from build123d import *

# Parameters (mm, degrees)
SKETCH1_R           = 5.55625
BOSS_EXTRUDE1_DEPTH = 3.175
SKETCH2_R           = 2.3876
CUT_EXTRUDE1_DEPTH  = 7.35


with BuildPart() as part:
    # Sketch1 → Boss-Extrude1 (new body, symmetric)
    with BuildSketch(Plane.XY):
        with BuildLine():
            Line((-88.9, 0), (-39.968180633, 0))
            ThreePointArc((-39.968180633, 0), (-38.358050091, 0.438559861), (-37.192731281, 1.633083694))
            Line((-37.192731281, 1.633083694), (-23.132268719, 26.941916306))
            ThreePointArc((-23.132268719, 26.941916306), (-21.966949909, 28.136440139), (-20.356819367, 28.575))
            Line((-20.356819367, 28.575), (20.356819367, 28.575))
            ThreePointArc((20.356819367, 28.575), (21.966949909, 28.136440139), (23.132268719, 26.941916306))
            Line((23.132268719, 26.941916306), (37.192731281, 1.633083694))
            ThreePointArc((37.192731281, 1.633083694), (38.358050091, 0.438559861), (39.968180633, 0))
            Line((39.968180633, 0), (88.9, 0))
            Line((88.9, 0), (88.9, -19.05))
            Line((88.9, -19.05), (-88.9, -19.05))
            Line((-88.9, -19.05), (-88.9, 0))
        make_face()
        with Locations((0, 15.875)):
            Circle(SKETCH1_R, mode=Mode.SUBTRACT)
    extrude(amount=BOSS_EXTRUDE1_DEPTH, both=True)

    # Sketch2 → Cut-Extrude1 (cut, through all)
    with BuildSketch(Plane.XY.offset(3.175)):
        with Locations((-64.77, -11.049)):
            Circle(SKETCH2_R)
        with Locations((72.7456, -11.049)):
            Circle(SKETCH2_R)
    extrude(amount=-CUT_EXTRUDE1_DEPTH, mode=Mode.SUBTRACT)


solid = part.part
Build history of the part. All positions in model axes, mm. A direction names the side the tool comes from. Give positions to 0.01 mm unless a question says otherwise; leave off trailing zeros. Order: outer loops, then holes, each group sorted by start corner. A loop starts at its lowest first (then second) coordinate and runs counter-clockwise, first axis right, second up. Notation, with made-up numbers: M 64.5,-36 L 117.5,-36 A28 ccw 117.5,-8 Z; hole C 64.25,43 d1. An arc over 180 degrees is marked long. Use one line per item in the form item = value.
Q1. Slice it at A-A, the plane x = 0. Write the cut outline in (y, z) (3 decimals).
Conclusion:
outline = M -19.05,-3.175 L 10.319,-3.175 L 10.319,3.175 L -19.05,3.175 Z; M 21.431,-3.175 L 28.575,-3.175 L 28.575,3.175 L 21.431,3.175 Z
Q2. Which spindle directions (+Z, -Z, +X, -X, +Y, -Y) get a long thin tool onto all of the face, cutting with end or side? Do faces 5 (the flat face through (64, 0, 0)), 6 (the flat face through (1, -19.05, 0)), 7 (the flat face through (-65, 0, 0)). Say none if no direction does.
Conclusion:
face_5 = +Z, -Z, +X, +Y
face_6 = +Z, -Z, +X, -X, -Y
face_7 = +Z, -Z, -X, +Y
Q3. Slice it at B-B, the plane z = -1.5. State how many separate pieces and enclosed holes the cut face has, and give its area (3 significant figures).
Conclusion:
separate_pieces = 1
enclosed_holes = 3
area = 4,980 mm2
Q4. Pin check, flat tips, straight feed: P1, Ø4, axis at x = -64.77, y = -11.049, coming from the -Z side; P2, Ø1, axis at y = 6, z = 1.5, coming from the +X side; P3, Ø1.9, axis at x = 76, z = -0.5, coming from the +Y side. Stop position of each tip, or through.
Conclusion:
P1 = through
P2 = 35.04
P3 = 0
Q5. Wall check: probe 1 along Y at (x, z) = (0, 0.5) (3 decimals); probe 2 along X at (y, z) = (-12, -0.75); probe 3 along Y at (x, z) = (-51, -0.5). Give the ranges that are in metal, low to high.
Conclusion:
probe_1 = -19.05 to 10.319, 21.431 to 28.575
probe_2 = -88.9 to -66.96, -62.58 to 70.56, 74.94 to 88.9
probe_3 = -19.05 to 0
Q6. Pull direction Y, two halves, no side cores. Call faces 1 (the cylindrical face through (-21.987, 28.124, 0.044)), 2 (the cylindrical face through (74.951, -11.963, 0.044)), 3 (the flat face through (88.9, -9, 0)), 4 (the cylindrical face through (-67.155, -10.944, 0.044)): released by +Y, released by -Y, zero draft, split by the parting line, or undercut.
Conclusion:
face_1 = released by +Y
face_2 = undercut
face_3 = zero draft
face_4 = undercut
